from build123d import *

# Parameters (mm, degrees)
SKETCH1_W                  = 122
SKETCH1_H                  = 96
BOSS_EXTRUDE1_DEPTH        = 2
F_3_5_3_5_DIAMETER_HOLE1_D = 3.5
FILLET1_R                  = 5


with BuildPart() as part:
    # Sketch1 → Boss-Extrude1 (new body)
    with BuildSketch(Plane.XY):
        with Locations((-39, 41)):
            Rectangle(SKETCH1_W, SKETCH1_H)
    extrude(amount=BOSS_EXTRUDE1_DEPTH)

    # Ø3.5 (3.5) Diameter Hole1 (through all)
    with Locations(Plane.XY.offset(2)):
        with Locations((0, 0), (15, 82), (-93, 82), (-93, 22)):
            Hole(F_3_5_3_5_DIAMETER_HOLE1_D / 2)

    # Fillet1
    fillet1_edges = [part.edges().sort_by_distance(p)[0] for p in [
        (-100, 89, 1),
        (22, 89, 1),
        (22, -7, 1),
        (-100, -7, 1),
    ]]
    fillet(fillet1_edges, radius=FILLET1_R)


solid = part.part
The listing builds one solid part. Answer for the finished solid, in the listing's coordinates (mm). Coordinates: 2 decimals unless noted, no trailing zeros. Loops run counter-clockwise (first coordinate to the right, second up) from the corner with the lowest first, then second, coordinate; pieces in that order, holes last. Notation, with made-up numbers: (-11, -15) -> (22, -15) arc R20 cw to (22, 11) -> close; hole circle Ø7 at (50.5, 46.5). An arc over 180 degrees is marked (long way). Write item = value, one per line. Start each with the question number.
1) A cutting plane is placed at B-B (y = 82). Give the vertices of the cut face in (x, z), then the cut area to 3 significant figures.
2) The mould has two halves that part along X. Classify faces 1 (the face through (-92.772, 23.735, 0.986)), 2 (the face through (-40, 42, 2)), 3 (the face through (20, -6, 1)): released by +X, released by -X, zero draft, split by the parting line, or undercut.
3) A cutting plane is placed at A-A (x = 15). Give the vertices of the cut face in (y, z).
4) Straight lines are drawn through the part: line 1 (X direction, y = 82, z = 1.2); line 2 (Y direction, x = -93, z = 1.45); line 3 (Y direction, x = 0, z = 1.25). For each, find the intervals that lie inside material, in ascending order. Write a range as from..to.
5) Given pin 1 Ø3 at (x, y) = (0, 0) entering from -Z, flat-ended and moving along its own axis, determine where the tip first touches the part or whether it passes through.
6) A cutting plane is placed at D-D (x = -93). Give the vertices of the cut face in (y, z).
7) A cutting plane is placed at C-C (y = 22). Give the vertices of the cut face in (x, z), then the cut area to 3 significant figures.
Responses:
q1.outline = (-100, 0) -> (-94.75, 0) -> (-94.75, 2) -> (-100, 2) -> close; (-91.25, 0) -> (13.25, 0) -> (13.25, 2) -> (-91.25, 2) -> close; (16.75, 0) -> (22, 0) -> (22, 2) -> (16.75, 2) -> close
q1.area = 230 mm²
q2.face_1 = undercut
q2.face_2 = zero draft
q2.face_3 = released by +X
q3.outline = (-7, 0) -> (80.25, 0) -> (80.25, 2) -> (-7, 2) -> close; (83.75, 0) -> (89, 0) -> (89, 2) -> (83.75, 2) -> close
q4.line_1 = -100..-94.75, -91.25..13.25, 16.75..22
q4.line_2 = -7..20.25, 23.75..80.25, 83.75..89
q4.line_3 = -7..-1.75, 1.75..89
q5.pin_1 = through
q6.outline = (-7, 0) -> (20.25, 0) -> (20.25, 2) -> (-7, 2) -> close; (23.75, 0) -> (80.25, 0) -> (80.25, 2) -> (23.75, 2) -> close; (83.75, 0) -> (89, 0) -> (89, 2) -> (83.75, 2) -> close
q7.outline = (-100, 0) -> (-94.75, 0) -> (-94.75, 2) -> (-100, 2) -> close; (-91.25, 0) -> (22, 0) -> (22, 2) -> (-91.25, 2) -> close
q7.area = 237 mm²
